Geometry: final body of the model. Coordinates: model frame, mm. A direction names the side the tool comes from. Give positions to 0.01 mm unless a question says otherwise; leave off trailing zeros. Write each loop counter-clockwise with the first axis right and the second up, starting at its lowest first coordinate (ties: lowest second). Pieces come first, ordered by that corner, then holes.
Q1. Cut plane B-B on x = -7.75. Return the cut outline in (y, z), plus the area to 3 significant figures.
Q2. Draft query along X for faces 4 (the face through (13.5, 0.17, 0.57)), 5 (the face through (10.579, 12.345, 49.268)), 6 (the face through (0.17, -13.53, 0.6)). Return one class per face: pulls with the +X half, pulls with the -X half, needs draft (parallel to the pull), parting line crosses it, or undercut.
Q3. Pin query (flat end, axial travel): pin 1 (1.5 mm diameter, centred on x = 11.5, y = 11.5, fed in from +Z); pin 2 (2 mm diameter, centred on x = -11.5, y = 11, fed in from +Z); pin 3 (6.5 mm diameter, centred on x = 4, y = -5, fed in from +Z). Return the tip coordinate at first contact, or that it passes through.
Q4. Cut plane D-D on x = 0. Return the cut outline in (y, z).
Q5. Cut plane C-C on y = -7. Return the cut outline in (x, z).
Q6. Line query: L1, parallel to Y at x = -11.5, z = 49.35; L2, parallel to Z at x = 5.25, y = 5; L3, parallel to Z at x = 10.25, y = -7. Output: solid intervals per line, ascending.
Q7. Cut plane A-A on y = 0. Return the cut outline in (x, z).
Q8. Reachability of faces 1 (the face through (0, 2, 63)), 2 (the face through (-12, 12, 48)), 3 (the face through (13.5, 13.53, 26.59)) from +Z, -Z, +X, -X, +Y, -Y: full face, straight path, thin tool, end or side. Return the list, or none.
```python
from build123d import *

# Parameters (mm, degrees)
SKETCH1_W           = 28.2
SKETCH1_H           = 28.2
BOSS_EXTRUDE1_DEPTH = 50.5
SKETCH2_R           = 11
BOSS_EXTRUDE2_DEPTH = 2
SKETCH3_R           = 2.5
BOSS_EXTRUDE3_DEPTH = 18
SKETCH4_W           = 15
SKETCH4_H           = 0.5
CUT_EXTRUDE1_DEPTH  = 5
SKETCH5_R           = 1.25
CUT_EXTRUDE2_DEPTH  = 2.5
FILLET1_R           = 2


with BuildPart() as part:
    # Sketch1 → Boss-Extrude1 (new body)
    with BuildSketch(Plane.XY):
        Rectangle(SKETCH1_W, SKETCH1_H)
    extrude(amount=BOSS_EXTRUDE1_DEPTH)

    # Sketch2 → Boss-Extrude2 (add)
    with BuildSketch(Plane.XY.offset(50.5)):
        with Locations(Location((0, 0, 0), (0, 0, 180))):
            Circle(SKETCH2_R)
    extrude(amount=BOSS_EXTRUDE2_DEPTH)

    # Sketch3 → Boss-Extrude3 (add)
    with BuildSketch(Plane.XY.offset(52.5)):
        Circle(SKETCH3_R)
    extrude(amount=BOSS_EXTRUDE3_DEPTH)

    # Sketch4 → Cut-Extrude1 (cut, symmetric)
    with BuildSketch(Plane(origin=(0, 0, 0), x_dir=(0, 0, -1), z_dir=(1, 0, 0))):
        with Locations((-63, 2.25)):
            Rectangle(SKETCH4_W, SKETCH4_H)
    extrude(amount=CUT_EXTRUDE1_DEPTH, both=True, mode=Mode.SUBTRACT)

    # Sketch5 → Cut-Extrude2 (cut)
    with BuildSketch(Plane.XY.offset(50.5)):
        with Locations((-11.5, 11.5)):
            Circle(SKETCH5_R)
        with Locations((11.5, 11.5)):
            Circle(SKETCH5_R)
        with Locations((11.5, -11.5)):
            Circle(SKETCH5_R)
        with Locations((-11.5, -11.5)):
            Circle(SKETCH5_R)
    extrude(amount=-CUT_EXTRUDE2_DEPTH, mode=Mode.SUBTRACT)

    # Fillet1
    fillet1_edges = [part.edges().sort_by_distance(p)[0] for p in [
        (0, -14.1, 0),
        (-14.1, 0, 0),
        (0, 14.1, 0),
        (14.1, 0, 0),
        (14.1, -14.1, 25.25),
        (-14.1, -14.1, 25.25),
        (-14.1, 14.1, 25.25),
        (14.1, 14.1, 25.25),
    ]]
    fillet(fillet1_edges, radius=FILLET1_R)


solid = part.part
```
Data:
1. outline: (-14.1, 2) arc R2 ccw to (-12.1, 0) - (12.1, 0) arc R2 ccw to (14.1, 2) - (14.1, 50.5) - (7.81, 50.5) - (7.81, 52.5) - (-7.81, 52.5) - (-7.81, 50.5) - (-14.1, 50.5) - close
1. area: 1,450 mm2
2. face 4: pulls with the +X half
2. face 5: undercut
2. face 6: needs draft
3. pin 1: stops at z = 48
3. pin 2: stops at z = 50.5
3. pin 3: stops at z = 52.5
4. outline: (-14.1, 2) arc R2 ccw to (-12.1, 0) - (12.1, 0) arc R2 ccw to (14.1, 2) - (14.1, 50.5) - (11, 50.5) - (11, 52.5) - (2.5, 52.5) - (2.5, 55.5) - (2, 55.5) - (2, 70.5) - (-2.5, 70.5) - (-2.5, 52.5) - (-11, 52.5) - (-11, 50.5) - (-14.1, 50.5) - close
5. outline: (-14.1, 2) arc R2 ccw to (-12.1, 0) - (12.1, 0) arc R2 ccw to (14.1, 2) - (14.1, 50.5) - (8.49, 50.5) - (8.49, 52.5) - (-8.49, 52.5) - (-8.49, 50.5) - (-14.1, 50.5) - close
6. L1: y = -14.1 to -12.75, -10.25 to 10.25, 12.75 to 14.1
6. L2: z = 0 to 52.5
6. L3: z = 0 to 50.5
7. outline: (-14.1, 2) arc R2 ccw to (-12.1, 0) - (12.1, 0) arc R2 ccw to (14.1, 2) - (14.1, 50.5) - (11, 50.5) - (11, 52.5) - (2.5, 52.5) - (2.5, 70.5) - (-2.5, 70.5) - (-2.5, 52.5) - (-11, 52.5) - (-11, 50.5) - (-14.1, 50.5) - close
8. face 1: +Z, +X, -X, +Y
8. face 2: +Z
8. face 3: +Z, -Z, +X, +Y
